Verification items for this drawing (mm, ordinates from the low corner). A direction names the side the tool comes from. Coordinates: 2 decimals unless noted, no trailing zeros. Order: outer loops, then holes, each group sorted by start corner. A loop starts at its lowest first (then second) coordinate and runs counter-clockwise, first axis right, second up. Notation, with made-up numbers: M 36.5,-13 L 88.5,-13 A14 cw 88.5,4 Z; hole C -12,73 d6. An arc over 180 degrees is marked long. One line per item, written item: value. Start each with the question number.
1) Access from +Z, -Z, +X, -X, +Y, -Y to the whole of each face (thin tool, end or side, straight path). Record for the marked faces 4 and 5.
2) Thickness scan on L1, parallel to Y at x = 1.5, z = 5; L2, parallel to Y at x = 5.25, z = 5; L3, parallel to Y at x = 3, z = 5. Record the ranges inside material, lowest first. Write a range as from..to.
3) Sectioned sample at C-C, the plane z = 5. Enter the section's corners in (x, y), then the cut area to 3 significant figures.
4) Sectioned sample at B-B, the plane x = 2. Enter the section's corners in (y, z).
5) Sectioned sample at A-A, the plane y = 24.5. Enter the section's corners in (x, z).
6) Go/stop test with a flat-tipped pin: P1, Ø2.5, axis at y = 24.5, z = 5, coming from the +X side. Record where the tip stops, or that it passes through.
7) Draft check along Y on the marked faces 1, 2 and 3. Enter one of: pulls with the +Y half, pulls with the -Y half, needs draft (parallel to the pull), parting line crosses it, or undercut.
8) Sectioned sample at D-D, the plane x = 3.5. Enter the section's corners in (y, z).
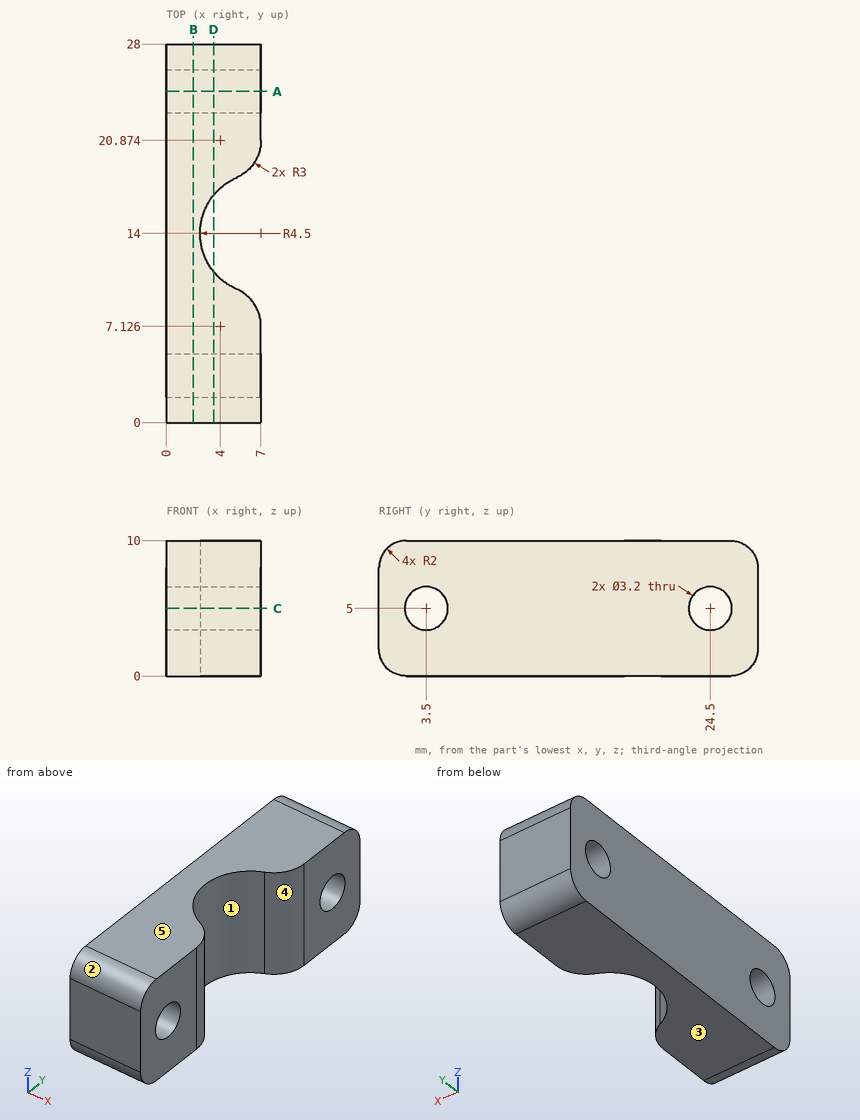
Final values:
1. face 4: +Z, -Z, +X
1. face 5: +Z, +X, -X, +Y, -Y
2. L1: y = 0..1.9, 5.1..22.9, 26.1..28
2. L2: y = 0..1.9, 5.1..9.85, 18.15..22.9, 26.1..28
2. L3: y = 0..1.9, 5.1..11.94, 16.06..22.9, 26.1..28
3. outline: M 0,0 L 7,0 L 7,1.9 L 0,1.9 Z; M 0,5.1 L 7,5.1 L 7,7.13 A3 ccw 5.2,9.88 A4.5 cw 5.2,18.12 A3 ccw 7,20.87 L 7,22.9 L 0,22.9 Z; M 0,26.1 L 7,26.1 L 7,28 L 0,28 Z
3. area: 118 mm^2
4. outline: M 0,2 A2 ccw 2,0 L 26,0 A2 ccw 28,2 L 28,8 A2 ccw 26,10 L 2,10 A2 ccw 0,8 Z; hole C 3.5,5 d3.2; hole C 24.5,5 d3.2
5. outline: M 0,0 L 7,0 L 7,3.4 L 0,3.4 Z; M 0,6.6 L 7,6.6 L 7,10 L 0,10 Z
6. P1: passes through
7. face 1: undercut
7. face 2: pulls with the -Y half
7. face 3: needs draft
8. outline: M 0,2 A2 ccw 2,0 L 11.17,0 L 11.17,10 L 2,10 A2 ccw 0,8 Z; M 16.83,0 L 26,0 A2 ccw 28,2 L 28,8 A2 ccw 26,10 L 16.83,10 Z; hole C 3.5,5 d3.2; hole C 24.5,5 d3.2
